CAD build for the part. Positions are in the model's coordinates, mm. A direction names the side the tool comes from. Round coordinates to 2 decimals unless told otherwise and drop trailing zeros. Write each loop counter-clockwise with the first axis right and the second up, starting at its lowest first coordinate (ties: lowest second). Pieces come first, ordered by that corner, then holes. Notation, with made-up numbers: (53.25, 44) - (68.25, 44) arc R18 cw to (68.25, 53) - close; hole circle Ø3 at (83.5, -25.5). An arc over 180 degrees is marked (long way). Use one line per item in the form item = value. Start each with the question number.
Item 1: Pull direction Z, two halves, no side cores. Call faces 3 (the flat face through (2, 126, 7)), 4 (the flat face through (14, -2, 3.175)), 5 (the cylindrical face through (1.565, -79.627, 14.992)): +Z half, -Z half, draft (parallel to the pull), parting line (faces both ways), or undercut.
Item 2: Pin check, flat tips, straight feed: pin 1 (10.5 mm diameter, centred on y = 82.8, z = 14.29, fed in from +X) (3 decimals); pin 2 (2 mm diameter, centred on y = -23.5, z = 22.5, fed in from -X); pin 3 (6.5 mm diameter, centred on x = 19, y = -0.5, fed in from +Z) (3 decimals). Stop position of each tip, or through.
Item 3: Band-saw the part on C-C, the plane x = 13. List the corners of the cut face in (y, z) (3 decimals), and give its area (3 significant figures).
Item 4: Band-saw the part on A-A, the plane y = 82.8. List the corners of the cut face in (x, z) (1 decimal).
Item 5: Band-saw the part on D-D, the plane z = 7.5. List the corners of the cut face in (x, y) (3 decimals), and give its area (3 significant figures).
Item 6: Band-saw the part on B-B, the plane y = 7.5. List the corners of the cut face in (x, z) (3 decimals), and give its area (3 significant figures).
Item 7: Tool access for faces 1 (the flat face through (0, -2, 13)), 2 (the flat face through (3.175, -2, 14)): list every direction of +Z, -Z, +X, -X, +Y, -Y with a clear straight run to the whole face (end or side of a thin tool).
Item 8: Drill centre lines: L1, parallel to Z at x = 2.55, y = 82.8; L2, parallel to X at y = 112, z = 5 (3 decimals). Where is each one in solid material? Low to high.
Autodesk Fusion 360 part; units mm, degrees
sketch "Sketch1" plane through (0, 0, 0) normal (0, 1, 0) x (1, 0, 0)
  line L0 (0, -25.4) -> (0, 0)
  line L1 (0, 0) -> (25.4, 0)
  line L2 (12.7, -12.7) -> (11.05, -11.05) construction
  line L3 (3.175, -25.4) -> (3.175, -3.175)
  line L4 (3.175, -3.175) -> (25.4, -3.175)
  line L5 (25.4, -3.175) -> (25.4, 0)
  line L6 (0, -25.4) -> (3.175, -25.4)
  dimension "d1" = 25.4
  dimension "d2" = 25.4
  dimension "d13" = 3.175
extrude "Extrude1" add sketch "Sketch1" along normal blind 126
hole "Hole3" at (3.175, 82.8, 14.2875) direction (-1, 0, 0) diameter 6.5 end through all
mirror "Mirror1" about plane through (0, 0, 0) normal (0, 1, 0) of bodies 1 merged
equation "d5 = ( 252 / 2 ) * 1 mm"
equation "d27 = ( 22.225 / 2 ) * 1 mm"
Determined:
q1.face_3 = draft
q1.face_4 = +Z half
q1.face_5 = undercut
q2.pin_1 = 3.175
q2.pin_2 = 0
q2.pin_3 = 3.175
q3.outline = (-126, 0) - (126, 0) - (126, 3.175) - (-126, 3.175) - close
q3.area = 800 mm²
q4.outline = (0, 0) - (25.4, 0) - (25.4, 3.2) - (3.2, 3.2) - (3.2, 11) - (0, 11) - close; (0, 17.5) - (3.2, 17.5) - (3.2, 25.4) - (0, 25.4) - close
q5.outline = (0, -126) - (3.175, -126) - (3.175, 126) - (0, 126) - close
q5.area = 800 mm²
q6.outline = (0, 0) - (25.4, 0) - (25.4, 3.175) - (3.175, 3.175) - (3.175, 25.4) - (0, 25.4) - close
q6.area = 151 mm²
q7.face_1 = +Z, -Z, -X, +Y, -Y
q7.face_2 = +Z, +X, +Y, -Y
q8.L1 = 0 to 11.04, 17.54 to 25.4
q8.L2 = 0 to 3.175
